Verification items for the finished model (mm, model axes). A direction names the side the tool comes from. Coordinates: 2 decimals unless noted, no trailing zeros. Write each loop counter-clockwise with the first axis right and the second up, starting at its lowest first coordinate (ties: lowest second). Pieces come first, ordered by that corner, then holes. Notation, with made-up numbers: (-37.5, 57) -> (-22.5, 57) arc R15 cw to (-22.5, 62) -> close; hole circle Ø9 at (2, -11). An arc over 180 degrees is marked (long way). Answer in a Markdown table with one row per item.
Autodesk Inventor part; units mm, degrees
ref_plane "YZ Plane" through (0, 0, 0) normal (1, 0, 0) x (0, 1, 0)
ref_plane "XZ Plane" through (0, 0, 0) normal (0, 1, 0) x (-1, 0, 0)
ref_plane "XY Plane" through (0, 0, 0) normal (0, 0, 1) x (1, 0, 0)
sketch "Эскиз1" plane through (0, 0, 0) normal (0, 0, 1) x (1, 0, 0)
  line L0 (-20.241, 29.4578) -> (24.759, 29.4578)
  line L1 (24.759, 29.4578) -> (24.759, -60.5422)
  line L2 (24.759, -60.5422) -> (-20.241, -60.5422)
  line L3 (-20.241, -60.5422) -> (-20.241, 29.4578)
  point P0 (0, 0)
  dimension "d0" = 90
  dimension "d1" = 45
extrude "Выдавливание1" add sketch "Эскиз1" along normal blind 2
sketch "Эскиз2" plane through (0, 0, 2) normal (0, 0, 1) x (1, 0, 0)
  line L0 (-20.241, 29.4578) -> (-20.241, -60.5422)
  line L1 (-20.241, -60.5422) -> (24.759, -60.5422)
  line L2 (-20.241, 29.4578) -> (-18.241, 29.4578)
  line L3 (-18.241, 29.4578) -> (-18.241, -60.5422)
  line L4 (-18.241, -60.5422) -> (-20.241, -60.5422)
  line L5 (-20.241, -60.5422) -> (-20.241, 29.4578)
  point P0 (0, 0)
  dimension "d4" = 2
extrude "Выдавливание2" add sketch "Эскиз2" along normal blind 28
sketch "Эскиз4" plane through (-20.241, 29.4578, 0) normal (0, 1, 0) x (1, 0, 0)
  line L0 (59.015, -17.4368) -> (44, -17.4368)
  line L1 (44, -17.4368) -> (44, 13.0776)
  line L2 (44, 13.0776) -> (59.015, 13.0776)
  line L3 (59.015, 13.0776) -> (59.015, -17.4368)
  line L4 (0, 0) -> (45, 0)
  point P0 (20.241, 0)
  point P1 (44, 0)
  point P2 (44, 0)
  point P3 (0, 0)
  dimension "d10" = 0
  dimension "d11" = 44
extrude "Выдавливание4" cut sketch "Эскиз4" against normal blind 1000
sketch "Эскиз5" plane through (-18.241, -60.5422, 2) normal (1, 0, 0) x (0, 0, -1)
  line L0 (2, 0) -> (-28, 0)
  line L1 (0, 90) -> (-28, 90)
  line L2 (-28, 0) -> (-26, 0)
  line L3 (-26, 0) -> (-26, 90)
  line L4 (-26, 90) -> (-28, 90)
  line L5 (-28, 90) -> (-28, 0)
  point P0 (2, 60.5422)
  point P1 (-26, 0)
  dimension "d14" = 2
extrude "Выдавливание5" add sketch "Эскиз5" along normal blind 42
sketch "Эскиз6" plane through (-18.241, -60.5422, 2) normal (1, 0, 0) x (0, 0, -1)
  circle A0 centre (-13, 80) radius 4
  line L0 (0, 90) -> (-26, 90)
  circle A1 centre (-13, 87) radius 1.5
  circle A2 centre (-20, 80) radius 1.5
  circle A3 centre (-13, 73) radius 1.5
  circle A4 centre (-6, 80) radius 1.5
  circle A5 centre (-13, 80) radius 7
  circle A6 centre (-13, 45) radius 4
  circle A7 centre (-20, 45) radius 1.5
  circle A8 centre (-13, 38) radius 1.5
  circle A9 centre (-6, 45) radius 1.5
  circle A10 centre (-13, 45) radius 7
  circle A11 centre (-13, 10) radius 4
  circle A12 centre (-20, 10) radius 1.5
  circle A13 centre (-13, 3) radius 1.5
  circle A14 centre (-6, 10) radius 1.5
  circle A15 centre (-13, 10) radius 7
  circle A16 centre (-13, 52) radius 1.5
  circle A17 centre (-13, 17) radius 1.5
  line L1 (2, 0) -> (-28, 0)
  line L2 (2, 90) -> (2, 0)
  point P0 (2, 60.5422)
  point P1 (-13, 90)
  point P2 (-13, 0)
  dimension "d17" = 8
  dimension "d19" = 0
  dimension "d21" = 14
  dimension "d22" = 3
  dimension "d23" = 3
  dimension "d24" = 3
  dimension "d25" = 3
  dimension "d26" = 0
  dimension "d27" = 0
  dimension "d28" = 7
  dimension "d29" = 7
  dimension "d30" = 0
  dimension "d31" = 7
  dimension "d32" = 0
  dimension "d33" = 7
  dimension "d34" = 8
  dimension "d35" = 14
  dimension "d36" = 3
  dimension "d37" = 3
  dimension "d38" = 3
  dimension "d39" = 0
  dimension "d40" = 0
  dimension "d41" = 7
  dimension "d42" = 7
  dimension "d43" = 0
  dimension "d44" = 7
  dimension "d45" = 0
  dimension "d46" = 7
  dimension "d47" = 8
  dimension "d48" = 14
  dimension "d49" = 3
  dimension "d50" = 3
  dimension "d51" = 3
  dimension "d52" = 0
  dimension "d53" = 0
  dimension "d54" = 7
  dimension "d55" = 7
  dimension "d56" = 0
  dimension "d57" = 7
  dimension "d58" = 0
  dimension "d59" = 7
  dimension "d60" = 3
  dimension "d61" = 3
  dimension "d65" = 17
  dimension "d67" = 10
  dimension "d68" = 21
  dimension "d69" = 15
  dimension "d70" = 15
extrude "Выдавливание6" cut sketch "Эскиз6" against normal blind 5 contours A0 | A1 A5 | A5 A1 | A5 A2 | A2 A5 | A5 A4 | A4 A5 | A5 A3 | A3 A5 | A6 | A7 A10 | A10 A7 | A16 A10 | A10 A16 | A10 A8 | A8 A10 | A10 A9 | A9 A10 | A11 | A12 A15 | A15 A12 | A17 A15 | A15 A17 | A15 A13 | A13 A15 | A15 A14 | A14 A15
sketch "Эскиз7" plane through (0, 0, 30) normal (0, 0, 1) x (1, 0, 0)
  circle A0 centre (11.759, 19.4578) radius 4
  circle A1 centre (11.759, 19.4578) radius 7
  circle A2 centre (4.759, 19.4578) radius 1.5
  circle A3 centre (11.759, 12.4578) radius 1.5
  circle A4 centre (18.759, 19.4578) radius 1.5
  circle A5 centre (11.759, 26.4578) radius 1.5
  line L0 (23.759, 29.4578) -> (23.759, -60.5422)
  line L1 (23.759, 29.4578) -> (-18.241, 29.4578)
  circle A6 centre (11.759, -15.5422) radius 4
  circle A7 centre (11.759, -15.5422) radius 7
  circle A8 centre (11.759, -22.5422) radius 1.5
  circle A9 centre (18.759, -15.5422) radius 1.5
  circle A10 centre (11.7213, -8.5423) radius 1.5
  circle A11 centre (11.759, -50.5422) radius 4
  circle A12 centre (11.759, -50.5422) radius 7
  circle A13 centre (11.759, -57.5422) radius 1.5
  circle A14 centre (18.759, -50.5422) radius 1.5
  circle A15 centre (11.759, -43.5422) radius 1.5
  line L2 (-20.241, -60.5422) -> (23.759, -60.5422)
  circle A16 centre (4.759, -15.5422) radius 1.5
  circle A17 centre (4.759, -50.5422) radius 1.5
  point P0 (0, 0)
  point P1 (23.759, 19.4578)
  point P2 (11.759, 29.4578)
  dimension "d73" = 8
  dimension "d74" = 14
  dimension "d75" = 3
  dimension "d76" = 3
  dimension "d77" = 3
  dimension "d78" = 3
  dimension "d80" = 0
  dimension "d81" = 12
  dimension "d82" = 0
  dimension "d83" = 0
  dimension "d84" = 7
  dimension "d85" = 0
  dimension "d86" = 7
  dimension "d87" = 7
  dimension "d88" = 8
  dimension "d89" = 14
  dimension "d91" = 3
  dimension "d92" = 3
  dimension "d93" = 3
  dimension "d94" = 0
  dimension "d95" = 7
  dimension "d96" = 0
  dimension "d97" = 7
  dimension "d98" = 7
  dimension "d99" = 8
  dimension "d100" = 14
  dimension "d102" = 3
  dimension "d103" = 3
  dimension "d104" = 3
  dimension "d105" = 0
  dimension "d106" = 7
  dimension "d107" = 0
  dimension "d108" = 7
  dimension "d109" = 7
  dimension "d110" = 0
  dimension "d111" = 0
  dimension "d112" = 0
  dimension "d114" = 35
  dimension "d115" = 35
  dimension "d116" = 3
  dimension "d117" = 3
  dimension "d118" = 3
extrude "Выдавливание7" cut sketch "Эскиз7" against normal blind 100 contours A0 | A1 A4 | A1 A4 | A5 A1 | A1 A5 | A3 A1 | A1 A3 | A2 A1 | A1 A2 | A6 | A7 A9 | A7 A9 | A10 A7 | A7 A10 | A8 A7 | A7 A8 | A16 A7 | A7 A16 | A11 | A12 A14 | A12 A14 | A15 A12 | A12 A15 | A13 A12 | A12 A13 | A17 A12 | A12 A17
sketch "Эскиз8" plane through (0, 0, 30) normal (0, 0, 1) x (1, 0, 0)
  circle A0 centre (18.259, -2.0422) radius 1.5
  circle A1 centre (18.259, -29.0422) radius 1.5
  line L0 (-20.241, 29.4578) -> (23.759, 29.4578)
  line L1 (23.759, 29.4578) -> (23.759, -60.5422)
  point P0 (0, 0)
  dimension "d121" = 3
  dimension "d122" = 3
  dimension "d123" = 31.5
  dimension "d124" = 5.5
  dimension "d125" = 0
  dimension "d126" = 27
extrude "Выдавливание8" cut sketch "Эскиз8" against normal blind 100
fillet "Сопряжение1" radius 3 6 edges at (-20.241, -15.5422, 30) (23.759, 29.4578, 29) (23.759, 29.4578, 1) (23.759, -60.5422, 29) (23.759, -60.5422, 1) (-20.241, -15.5422, 0)
properties part number "основа" material "Сталь"
1. Sectioned sample at B-B, the plane z = 8. Record the cut outline in (x, y).
Findings below:
| item | result |
|---|---|
| outline | (-20.24, -60.54) -> (-18.24, -60.54) -> (-18.24, -52.04) -> (-20.24, -52.04) -> close; (-20.24, -49.04) -> (-18.24, -49.04) -> (-18.24, -17.04) -> (-20.24, -17.04) -> close; (-20.24, -14.04) -> (-18.24, -14.04) -> (-18.24, 17.96) -> (-20.24, 17.96) -> close; (-20.24, 20.96) -> (-18.24, 20.96) -> (-18.24, 29.46) -> (-20.24, 29.46) -> close |
2. Material ranges on probe 1 along Z at (x, y) = (-8.5, 4); probe 2 along X at (y, z) = (-6.5, 24.25), recorded low to high. Write a range as from..to.
Findings below:
| item | result |
|---|---|
| probe 1 | z = 0..2, 28..30 |
| probe 2 | x = -20.24..-18.24 |
3. Go/stop test with flat-tipped pins: pin 1 (6 mm diameter, centred on y = -25, z = 8, fed in from +X); pin 2 (1.8 mm diameter, centred on x = 4.76, y = -50.54, fed in from -Z). Record where each tip stops, or that it passes through.
Findings below:
| item | result |
|---|---|
| pin 1 | stops at x = -18.24 |
| pin 2 | passes through |
4. Sectioned sample at A-A, the plane x = -7.5. Record the cut outline in (y, z).
Findings below:
| item | result |
|---|---|
| outline | (-60.54, 0) -> (29.46, 0) -> (29.46, 2) -> (-60.54, 2) -> close; (-60.54, 28) -> (29.46, 28) -> (29.46, 30) -> (-60.54, 30) -> close |
5. Release check for a two-part mould opening along X. For faces 1 (the face through (3, -15, 0)), 2 (the face through (11.4, -59, 29)), 3 (the face through (22.857, -59.687, 1.014)) record: released by +X, released by -X, zero draft, split by the parting line, or undercut.
Findings below:
| item | result |
|---|---|
| face 1 | zero draft |
| face 2 | undercut |
| face 3 | released by +X |
6. Sectioned sample at C-C, the plane z = 12.5. Record the cut outline in (x, y).
Findings below:
| item | result |
|---|---|
| outline | (-20.24, -60.54) -> (-18.24, -60.54) -> (-18.24, -53.66) -> (-20.24, -53.66) -> close; (-20.24, -47.42) -> (-18.24, -47.42) -> (-18.24, -18.66) -> (-20.24, -18.66) -> close; (-20.24, -12.42) -> (-18.24, -12.42) -> (-18.24, 16.34) -> (-20.24, 16.34) -> close; (-20.24, 22.58) -> (-18.24, 22.58) -> (-18.24, 29.46) -> (-20.24, 29.46) -> close |
7. Sectioned sample at D-D, the plane x = 11.5. Count the separate pieces of the cut face and the enclosed holes in it, and give its area (3 significant figures).
Findings below:
| item | result |
|---|---|
| separate pieces | 20 |
| enclosed holes | 0 |
| area | 193 mm² |
8. Access from +Z, -Z, +X, -X, +Y, -Y to the whole of each face (thin tool, end or side, straight path). Record for faces 4 (the face through (-18.241, -15, 6)), 5 (the face through (10.892, 15.553, 1.014)).
Findings below:
| item | result |
|---|---|
| face 4 | +X, +Y, -Y |
| face 5 | +Z, -Z |
